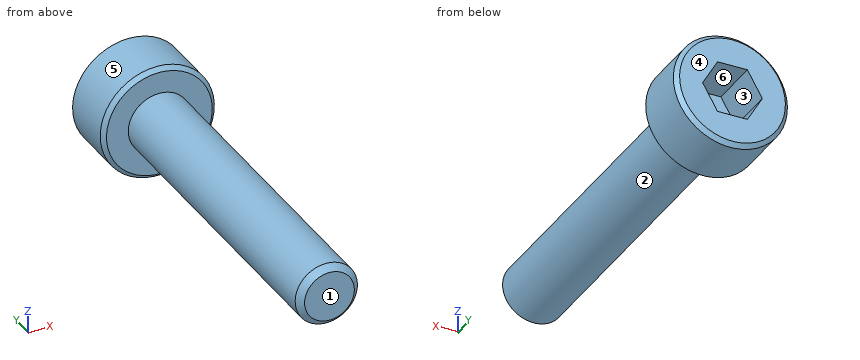
from build123d import *

# Parameters (mm, degrees)
CHAMFER_1_SIZE      = 0.2
CHAMFER_2_SIZE      = 0.3
CUT_EXTRUDE_1_DEPTH = 2.5


with BuildPart() as part:
    # 草图1 → 旋转1 (revolve)
    with BuildSketch(Plane.XY, mode=Mode.PRIVATE) as revolve_1_sk:
        Polygon((1.5, 0), (2.75, 0), (2.75, 3), (0, 3), (0, 0), (0, -16), (1.5, -16), align=None)
    revolve(revolve_1_sk.sketch.rotate(Axis((0, 3, 0), (0, -1, 0)), 90), axis=Axis((0, 3, 0), (0, -1, 0)))

    # 倒角1
    chamfer_1_edges = [part.edges().sort_by_distance(p)[0] for p in [
        (0, 3, -2.75),
        (0, 0, -2.75),
    ]]
    chamfer(chamfer_1_edges, length=CHAMFER_1_SIZE)

    # 倒角2
    chamfer_2_edges = [part.edges().sort_by_distance(p)[0] for p in [
        (0, -16, -1.5),
    ]]
    chamfer(chamfer_2_edges, length=CHAMFER_2_SIZE)

    # 草图2 → 切除-拉伸1 (cut)
    with BuildSketch(Plane(origin=(0, 3, 0), x_dir=(1, 0, 0), z_dir=(0, 1, 0))):
        Polygon((-0.72, 1.247076581), (0.72, 1.247076581), (1.44, 0), (0.72, -1.247076581), (-0.72, -1.247076581), (-1.44, 0), align=None)
    extrude(amount=-CUT_EXTRUDE_1_DEPTH, mode=Mode.SUBTRACT)


solid = part.part
Part model, mm, in its own coordinate system. Face numbers are marked on the shaded views. A direction names the side the tool comes from. Coordinates: 2 decimals unless noted, no trailing zeros. Order: outer loops, then holes, each group sorted by start corner. A loop starts at its lowest first (then second) coordinate and runs counter-clockwise, first axis right, second up. Notation, with made-up numbers: M -14.75,-33.75 L 42.25,-33.75 A15 ccw 42.25,-18.75 Z; hole C 52.25,37 d9. An arc over 180 degrees is marked long. One line per question, with ' | ' between items.
Q1. Slice it at A-A (y = 1.5). Give the cut face in (x, z), and give its area (3 significant figures).
A:
outline: C 0,0 d5.5; hole M -1.44,0 L -0.72,-1.25 L 0.72,-1.25 L 1.44,0 L 0.72,1.25 L -0.72,1.25 Z | area: 18.4 mm^2
Q2. Slice it at C-C (y = -2.5). Give the cut face in (x, z), and give its area (3 significant figures).
A:
outline: C 0,0 d3 | area: 7.07 mm^2
Q3. Pin check, flat tips, straight feed: P1, Ø2, axis at y = -8, z = -0.5, coming from the +X side; P2, Ø1.2, axis at x = 0, z = 0, coming from the +Y side; P3, Ø3, axis at x = 0, y = -4, coming from the +Z side. Stop position of each tip, or through.
A:
P1: stops at x = 1.5 | P2: stops at y = 0.5 | P3: stops at z = 1.5
Q4. 3-axis set-ups, long thin cutter, end or side, ignore diameter. For the marked faces 1, 2 and 3: which of +Z, -Z, +X, -X, +Y, -Y reach the whole face in a straight line?
A:
face 1: +Z, -Z, +X, -X, -Y | face 2: -Y | face 3: +Y
Q5. Slice it at B-B (x = 0). Give the cut face in (y, z), and give its area (3 significant figures).
A:
outline: M -16,-1.2 L -15.7,-1.5 L 0,-1.5 L 0,-2.55 L 0.2,-2.75 L 2.8,-2.75 L 3,-2.55 L 3,-1.25 L 0.5,-1.25 L 0.5,1.25 L 3,1.25 L 3,2.55 L 2.8,2.75 L 0.2,2.75 L 0,2.55 L 0,1.5 L -15.7,1.5 L -16,1.2 Z | area: 58.1 mm^2
Q6. Two-plate mould, pull along X, no slides. Class the marked faces 4, 5 and 6: +X half, -X half, draft (parallel to the pull), parting line (faces both ways), or undercut.
A:
face 4: draft | face 5: parting line | face 6: undercut
Q7. Drill centre lines: line 1 (Y direction, x = -1.35, z = 1.05); line 2 (Y direction, x = 0.3, z = -1.05); line 3 (X direction, y = 2, z = -1.05). Where is each one in solid material? Low to high.
A:
line 1: y = 0 to 3 | line 2: y = -16 to 0.5 | line 3: x = -2.54 to -0.83, 0.83 to 2.54
